```python
from build123d import *

# Parameters (mm, degrees)
F0_W     = 33.5
F0_H     = 28
F1_DEPTH = 3
F2_R     = 2
F3_W     = 2.9
F3_H     = 15
F4_DEPTH = 4
F5_W     = 12.03
F5_H     = 1.51
F6_DEPTH = 0.6
F7_R     = 2


# Not quite as in the source:
# - a pattern or mirror of a feature is missing from the dataset's text; its kind, count and spacing are read off the source's solid


with BuildPart() as f1:
    # F0 (on Top) → F1 (new body)
    with BuildSketch(Plane.XY):
        Rectangle(F0_W, F0_H)
    extrude(amount=F1_DEPTH)

    # F2
    f2_edges = [f1.edges().sort_by_distance(p)[0] for p in [
        (-16.75, -14, 1.5),
        (16.75, -14, 1.5),
        (16.75, 14, 1.5),
        (-16.75, 14, 1.5),
    ]]
    fillet(f2_edges, radius=F2_R)

    # F3 (on face) → F4 (join)
    with BuildSketch(Plane.XY.offset(3)):
        with Locations((15.3, 0)):
            Rectangle(F3_W, F3_H)
    f4 = extrude(amount=F4_DEPTH)

    # F4_copies: F4 across plane
    add(f4.mirror(Plane(origin=(0, 0, 0), x_dir=(0, 0, -1), z_dir=(-1, 0, 0))))

    # F5 (on face) → F6 (cut)
    with BuildSketch(Plane(origin=(13.85, 0, 0), x_dir=(0, -1, 0), z_dir=(-1, 0, 0))):
        with Locations((0, 3.755)):
            Rectangle(F5_W, F5_H)
    f6 = extrude(amount=-F6_DEPTH, mode=Mode.SUBTRACT)

    # F6_copies: F6 across plane
    add(f6.mirror(Plane(origin=(0, 0, 0), x_dir=(0, 0, -1), z_dir=(-1, 0, 0))), mode=Mode.SUBTRACT)

    # F7
    f7_edges = [f1.edges().sort_by_distance(p)[0] for p in [
        (15.3, 7.5, 7),
        (15.3, -7.5, 7),
        (-15.3, 7.5, 7),
        (-15.3, -7.5, 7),
    ]]
    fillet(f7_edges, radius=F7_R)


solid = f1.part
```
CAD build for the part. Positions are in the model's coordinates, mm. A direction names the side the tool comes from. Coordinates: 2 decimals unless noted, no trailing zeros. Write each loop counter-clockwise with the first axis right and the second up, starting at its lowest first coordinate (ties: lowest second). Pieces come first, ordered by that corner, then holes. Notation, with made-up numbers: (-30.5, 3.5) -> (-13.5, 3.5) arc R29 ccw to (-13.5, 27.5) -> close; hole circle Ø1 at (13, 26.25). An arc over 180 degrees is marked (long way). Return JSON: item names as keys, results as strings. Group by question number.
Q1. Pull direction Z, two halves, no side cores. Call faces 1 (the face through (14.45, 0, 4)), 2 (the face through (15.32, 6.93, 6.4)), 3 (the face through (-15, -7.5, 4)), 4 (the face through (0, 0, 0)): released by +Z, released by -Z, zero draft, split by the parting line, or undercut.
Q2. Drill centre lines: line 1 (X direction, y = 5, z = 4.75); line 2 (X direction, y = 0.5, z = 4.25); line 3 (Z direction, x = -6, y = -9). Where is each one in solid material? Low to high.
Q3. Cut at A-A, the plane y = 1.5. Give the cut face in (x, z).
Q4. Cut at D-D, the plane y = -7. Give the cut face in (x, z).
Q5. Cut at B-B, the plane z = 6.5. Give the cut face in (x, y).
Q6. Which spindle directions (+Z, -Z, +X, -X, +Y, -Y) get a long thin tool onto all of the face, cutting with end or side? Do faces 5 (the face through (15, -7.5, 4)), 6 (the face through (13.85, 0, 5)), 7 (the face through (15, 7.5, 4)). Say none if no direction does.
Q7. Flat gauge pins, fed straight in: pin 1 (1.6 mm diameter, centred on x = 15, z = 4.5, fed in from +Y); pin 2 (1.6 mm diameter, centred on x = 15.5, z = 3.5, fed in from -Y); pin 3 (12 mm diameter, centred on x = 3.5, y = 7, fed in from +Z). Where does each tip first touch, or does it go through?
Q8. Cut at C-C, the plane x = -13. Give the cut face in (y, z).
Returned:
{
 "1": {"face 1": "undercut", "face 2": "released by +Z", "face 3": "zero draft", "face 4": "released by -Z"},
 "2": {"line 1": "x = -16.75 to -13.85, 13.85 to 16.75", "line 2": "x = -16.75 to -14.45, 14.45 to 16.75", "line 3": "z = 0 to 3"},
 "3": {"outline": "(-16.75, 0) -> (16.75, 0) -> (16.75, 7) -> (13.85, 7) -> (13.85, 4.51) -> (14.45, 4.51) -> (14.45, 3) -> (-14.45, 3) -> (-14.45, 4.51) -> (-13.85, 4.51) -> (-13.85, 7) -> (-16.75, 7) -> close"},
 "4": {"outline": "(-16.75, 0) -> (16.75, 0) -> (16.75, 6.32) -> (13.85, 6.32) -> (13.85, 3) -> (-13.85, 3) -> (-13.85, 6.32) -> (-16.75, 6.32) -> close"},
 "5": {"outline": "(-16.75, -6.82) -> (-13.85, -6.82) -> (-13.85, 6.82) -> (-16.75, 6.82) -> close; (13.85, -6.82) -> (16.75, -6.82) -> (16.75, 6.82) -> (13.85, 6.82) -> close"},
 "6": {"face 5": "+Z, +X, -X, -Y", "face 6": "+Z, +Y, -Y", "face 7": "+Z, +X, -X, +Y"},
 "7": {"pin 1": "stops at y = 7.5", "pin 2": "stops at y = -14", "pin 3": "stops at z = 3"},
 "8": {"outline": "(-14, 0) -> (14, 0) -> (14, 3) -> (-14, 3) -> close"}
}
